Input: part model. Units: mm. Frame: model coordinates. Face numbers are marked on the shaded views. A direction names the side the tool comes from. Round coordinates to 2 decimals unless told otherwise and drop trailing zeros. Loops run counter-clockwise (first coordinate to the right, second up) from the corner with the lowest first, then second, coordinate; pieces in that order, holes last. Notation, with made-up numbers: (83.25, -32.5) -> (95.25, -32.5) arc R18 cw to (95.25, -24.5) -> close; hole circle Ø6 at (16.5, -5). An arc over 180 degrees is marked (long way). Answer in a Markdown table with one row per item. Add a question column.
Q1. Reachability of the marked faces 1 and 2 from +Z, -Z, +X, -X, +Y, -Y: full face, straight path, thin tool, end or side. Return the list, or none.
Q2. Section D-D, the plane z = -11.5. Output: boundary loops of the cut face in (x, y), and give its area (3 significant figures).
Q3. Pin query (flat end, axial travel): pin 1 (1 mm diameter, centred on x = -4.5, z = -3, fed in from -Y). Return the tip coordinate at first contact, or that it passes through.
Q4. Section A-A, the plane y = -15. Output: boundary loops of the cut face in (x, z).
Q5. Ray query, L1, parallel to Z at x = -24.25, y = -15; L2, parallel to X at y = -27, z = 15; L3, parallel to Y at x = 26.75, z = -25. Return the intervals inside material, ascending. Write a range as from..to.
Q6. Section C-C, the plane x = 29. Output: boundary loops of the cut face in (y, z).
Q7. Mould query, pull axis Z, two halves, no side actions, for the marked faces 3, 4 and 5. Classes: pulls with the +Z half, pulls with the -Z half, needs draft (parallel to the pull), parting line crosses it, or undercut.
Q8. Section B-B, the plane z = 25. Output: boundary loops of the cut face in (x, y), and give its area (3 significant figures).
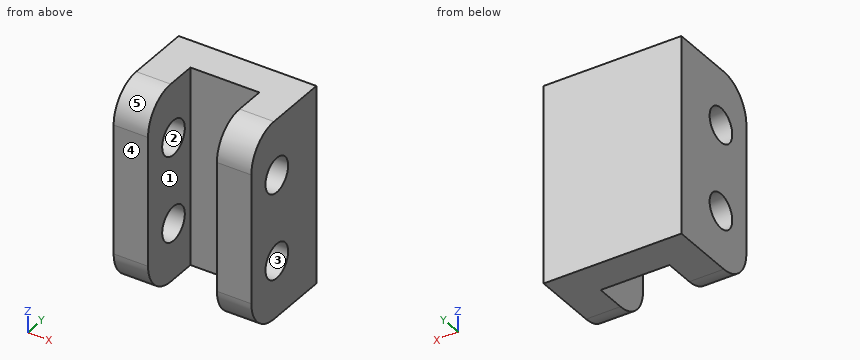
Autodesk Inventor part; units mm, degrees
ref_plane "YZ Plane" through (0, 0, 0) normal (1, 0, 0) x (0, 1, 0)
ref_plane "XZ Plane" through (0, 0, 0) normal (0, 1, 0) x (-1, 0, 0)
ref_plane "XY Plane" through (0, 0, 0) normal (0, 0, 1) x (1, 0, 0)
sketch "Sketch1" plane through (0, 0, 0) normal (0, 1, 0) x (-1, 0, 0)
  line L0 (40, 57.5) -> (-40, 57.5)
  line L1 (-40, 57.5) -> (-40, -57.5)
  line L2 (-40, -57.5) -> (40, -57.5)
  line L3 (40, -57.5) -> (40, 57.5)
  point P0 (0, 0)
  point P1 (40, 0)
  point P2 (0, 57.5)
  dimension "d0" = 115
  dimension "d1" = 80
extrude "Extrusion1" add sketch "Sketch1" along normal blind 20
sketch "Sketch12" plane through (0, 0, 0) normal (0, -1, 0) x (1, 0, 0)
  line L0 (-40, 57.5) -> (-20, 57.5)
  line L1 (-20, 57.5) -> (-20, -57.5)
  line L2 (-20, -57.5) -> (-40, -57.5)
  line L3 (-40, -57.5) -> (-40, 57.5)
  line L4 (-40, -57.5) -> (-40, 57.5)
  line L5 (0, 100.8809) -> (0, -116.5773) construction
  line L6 (40, 57.5) -> (20, 57.5)
  line L7 (20, 57.5) -> (20, -57.5)
  line L8 (20, -57.5) -> (40, -57.5)
  line L9 (40, -57.5) -> (40, 57.5)
  point P0 (0, 0)
  point P1 (-40, 0)
  point P2 (0, 0)
  point P3 (-20, 0)
  dimension "d56" = 20
  dimension "d57" = 115
extrude "Extrusion11" add sketch "Sketch12" along normal blind 37.5
sketch "Sketch13" plane through (-40, 0, 57.5) normal (-1, 0, 0) x (0, 0, 1)
  line L0 (0, 0) -> (-115, 0)
  point P0 (-57.5, 0)
  point P1 (-32.5, -15)
  point P2 (-82.5, -15)
  point P3 (-57.5, -15)
  point P4 (-57.5, 0)
  dimension "d129" = 25
  dimension "d130" = 25
  dimension "d131" = 15
hole "Hole2" at (-40, -15, 25) at (-40, -15, -25) direction (1, 0, 0) diameter 20 end through all
fillet "Fillet19" radius 20 4 edges at (-30, -37.5, -57.5) (30, -37.5, -57.5) (30, -37.5, 57.5) (-30, -37.5, 57.5)
properties part number "Y_Slider_Part_mit_Schrittmotor"
Answer block:
| question | item | result |
|---|---|---|
| 1 | face 1 | +Z, -Z, -Y |
| 1 | face 2 | +X, -X |
| 2 | outline | (-40, -37.5) -> (-20, -37.5) -> (-20, 0) -> (20, 0) -> (20, -37.5) -> (40, -37.5) -> (40, 20) -> (-40, 20) -> close |
| 2 | area | 3,100 mm^2 |
| 3 | pin 1 | y = 0 |
| 4 | outline | (-40, -57.5) -> (-20, -57.5) -> (-20, -35) -> (-40, -35) -> close; (-40, -15) -> (-20, -15) -> (-20, 15) -> (-40, 15) -> close; (-40, 35) -> (-20, 35) -> (-20, 57.5) -> (-40, 57.5) -> close; (20, -57.5) -> (40, -57.5) -> (40, -35) -> (20, -35) -> close; (20, -15) -> (40, -15) -> (40, 15) -> (20, 15) -> close; (20, 35) -> (40, 35) -> (40, 57.5) -> (20, 57.5) -> close |
| 5 | L1 | -57.5..-35, -15..15, 35..57.5 |
| 5 | L2 | -40..-20, 20..40 |
| 5 | L3 | -37.5..-25, -5..20 |
| 6 | outline | (-37.5, -37.5) arc R20 ccw to (-17.5, -57.5) -> (20, -57.5) -> (20, 57.5) -> (-17.5, 57.5) arc R20 ccw to (-37.5, 37.5) -> close; hole circle Ø20 at (-15, -25); hole circle Ø20 at (-15, 25) |
| 7 | face 3 | undercut |
| 7 | face 4 | needs draft |
| 7 | face 5 | pulls with the +Z half |
| 8 | outline | (-40, -37.5) -> (-20, -37.5) -> (-20, -25) -> (-40, -25) -> close; (-40, -5) -> (-20, -5) -> (-20, 0) -> (20, 0) -> (20, -5) -> (40, -5) -> (40, 20) -> (-40, 20) -> close; (20, -37.5) -> (40, -37.5) -> (40, -25) -> (20, -25) -> close |
| 8 | area | 2,300 mm^2 |
